Part model, mm, in its own coordinate system. A direction names the side the tool comes from. Round coordinates to 2 decimals unless told otherwise and drop trailing zeros. Order: outer loops, then holes, each group sorted by start corner. A loop starts at its lowest first (then second) coordinate and runs counter-clockwise, first axis right, second up. Notation, with made-up numbers: (16, 64.5) - (31, 64.5) arc R21 ccw to (31, 100.5) - close; hole circle Ø3 at (39, -16). An arc over 180 degrees is marked (long way). Return JSON: item names as keys, results as strings. Group by question number.
Item 1: Tool access for faces 1 (the face through (54, 0, 5)), 2 (the face through (-12.9, -21.3, 46.1)), 3 (the face through (41.8, 0, 24)): list every direction of +Z, -Z, +X, -X, +Y, -Y with a clear straight run to the whole face (end or side of a thin tool).
Item 2: Saw through at A-A on y = 0. List the corners of the cut face in (x, z).
Item 3: Saw through at B-B on z = 8.5. List the corners of the cut face in (x, y), and give its area (3 significant figures).
Item 4: Probe probe 1 along Y at (x, z) = (1, 37); probe 2 along X at (y, z) = (0.5, 40); probe 3 along Z at (x, y) = (-38, -17.5). List the from-to ranges inside material, lowest first.
Item 5: Saw through at D-D on x = 48.5. List the corners of the cut face in (y, z), and give its area (3 significant figures).
Item 6: Saw through at C-C on x = 5. List the corners of the cut face in (y, z).
Item 7: Drop flat-ended pins along their axis: pin 1 (3 mm diameter, centred on y = -2.5, z = 6, fed in from +X); pin 2 (2 mm diameter, centred on x = -15, y = 1.5, fed in from +Z); pin 3 (2 mm diameter, centred on x = 46.5, y = -15, fed in from +Z). Give the stop position or say it passes through.
Item 8: Two-plate mould, pull along X, no slides. Class faces 4 (the face through (-42.14, -21.3, 23.37)), 5 (the face through (1, 22.2, 23)), 6 (the face through (57.27, 0.34, 2.46)), 7 (the face through (0, 0, 1.2)): released by +X, released by -X, zero draft, split by the parting line, or undercut.
```python
from build123d import *

# Parameters (mm, degrees)
SKETCH_1_W          = 86
SKETCH_1_H          = 44.4
EXTRUDE_1_DEPTH     = 46.1
EXTRUDE_2_DEPTH     = 5
SKETCH_3_W          = 83
SKETCH_3_H          = 42
CUT_EXTRUDE_1_DEPTH = 44.9
FILLET_1_R          = 3


with BuildPart() as part:
    # Эскиз1 → Бобышка-Вытянуть1 (new body)
    with BuildSketch(Plane.XY):
        Rectangle(SKETCH_1_W, SKETCH_1_H)
    extrude(amount=EXTRUDE_1_DEPTH)

    # Эскиз2 → Бобышка-Вытянуть2 (add)
    with BuildSketch(Plane.XY):
        with BuildLine():
            Line((43, 13.108775687), (43, 17.2))
            ThreePointArc((43, 17.2), (57.273546839, 0), (43, -17.2))
            Line((43, -17.2), (43, -13.108775687))
            ThreePointArc((43, -13.108775687), (53.273546839, 0), (43, 13.108775687))
        make_face()
    extrude(amount=EXTRUDE_2_DEPTH)

    # Эскиз3 → Вырез-Вытянуть1 (cut)
    with BuildSketch(Plane.XY.offset(46.1)):
        with Locations((0.3, 0)):
            Rectangle(SKETCH_3_W, SKETCH_3_H)
    extrude(amount=-CUT_EXTRUDE_1_DEPTH, mode=Mode.SUBTRACT)

    # Скругление1
    fillet_1_edges = [part.edges().sort_by_distance(p)[0] for p in [
        (-41.2, 21, 23.65),
        (-41.2, -21, 23.65),
        (-43, -22.2, 23.05),
        (-43, 22.2, 23.05),
    ]]
    fillet(fillet_1_edges, radius=FILLET_1_R)


solid = part.part
```
Filled in:
{
 "1": {"face 1": "+Z, +X, +Y, -Y", "face 2": "+Z, +X, -X, +Y, -Y", "face 3": "+Z"},
 "2": {"outline": "(-43, 0) - (43, 0) - (43, 46.1) - (41.8, 46.1) - (41.8, 1.2) - (-41.2, 1.2) - (-41.2, 46.1) - (-43, 46.1) - close; (53.27, 0) - (57.27, 0) - (57.27, 5) - (53.27, 5) - close"},
 "3": {"outline": "(-43, -19.2) arc R3 ccw to (-40, -22.2) - (43, -22.2) - (43, 22.2) - (-40, 22.2) arc R3 ccw to (-43, 19.2) - close; hole (-41.2, -18) arc R3 ccw to (-38.2, -21) - (41.8, -21) - (41.8, 21) - (-38.2, 21) arc R3 ccw to (-41.2, 18) - close", "area": "332 mm^2"},
 "4": {"probe 1": "y = -22.2 to -21, 21 to 22.2", "probe 2": "x = -43 to -41.2, 41.8 to 43", "probe 3": "z = 0 to 1.2"},
 "5": {"outline": "(-15.17, 0) - (-10.3, 0) - (-10.3, 5) - (-15.17, 5) - close; (10.3, 0) - (15.17, 0) - (15.17, 5) - (10.3, 5) - close", "area": "48.7 mm^2"},
 "6": {"outline": "(-22.2, 0) - (22.2, 0) - (22.2, 46.1) - (21, 46.1) - (21, 1.2) - (-21, 1.2) - (-21, 46.1) - (-22.2, 46.1) - close"},
 "7": {"pin 1": "stops at x = 57.22", "pin 2": "stops at z = 1.2", "pin 3": "stops at z = 5"},
 "8": {"face 4": "released by -X", "face 5": "zero draft", "face 6": "released by +X", "face 7": "undercut"}
}
